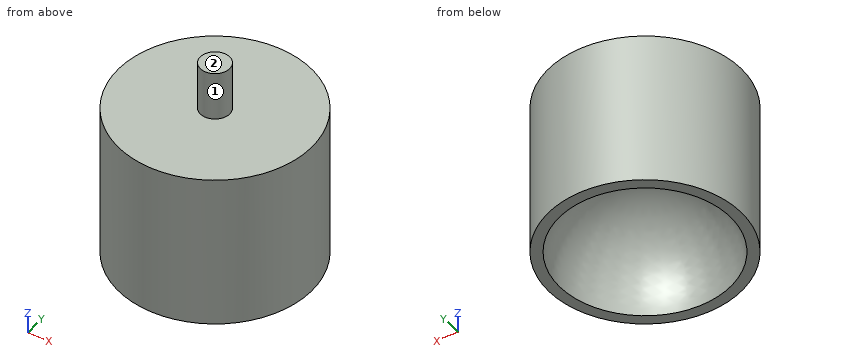
from build123d import *

# Parameters (mm, degrees)
F0_R     = 5.925
F1_DEPTH = 9.5
F2_R     = 0.9
F3_DEPTH = 3


with BuildPart() as f1:
    # F0 (on Top) → F1 (new body)
    with BuildSketch(Plane.XY):
        Circle(F0_R)
    extrude(amount=F1_DEPTH)

    # F2 (on face) → F3 (join)
    with BuildSketch(Plane.XY.offset(9.5)):
        Circle(F2_R)
    extrude(amount=F3_DEPTH)

    # F4 (on Front) → F5 (revolve, cut)
    with BuildSketch(Plane.XZ):
        with BuildLine():
            Line((0, 0), (5.25, 0))
            ThreePointArc((5.25, 0), (3.712311, 3.712311), (0, 5.25))
            Line((0, 5.25), (0, 0))
        make_face()
    revolve(axis=Axis((0, 0, 7.387147), (0, 0, 1)), mode=Mode.SUBTRACT)


solid = f1.part
Part model, mm, in its own coordinate system. Face numbers are marked on the shaded views. A direction names the side the tool comes from. Round coordinates to 2 decimals unless told otherwise and drop trailing zeros. Loops run counter-clockwise (first coordinate to the right, second up) from the corner with the lowest first, then second, coordinate; pieces in that order, holes last. Notation, with made-up numbers: (-3.5, 60.25) - (3.5, 60.25) arc R16 ccw to (3.5, 81.25) - close; hole circle Ø5 at (33, 54). An arc over 180 degrees is marked (long way). Answer as a JSON object with one key per item and string values.
Item 1: Band-saw the part on A-A on z = 6.5. List the corners of the cut face in (x, y) (3 decimals), plus the area to 3 significant figures.
Output:
{"outline": "circle Ø11.85 at (0, 0)", "area": "110 mm2"}
Item 2: Tool access for the marked faces 1 and 2: list every direction of +Z, -Z, +X, -X, +Y, -Y with a clear straight run to the whole face (end or side of a thin tool).
Output:
{"face 1": "+Z", "face 2": "+Z, +X, -X, +Y, -Y"}
Item 3: Pin check, flat tips, straight feed: pin 1 (2 mm diameter, centred on y = -3.5, z = 8, fed in from +X); pin 2 (4 mm diameter, centred on y = -2.5, z = 10.5, fed in from -X) (3 decimals); pin 3 (3 mm diameter, centred on x = 4.5, z = 9, fed in from +Y). Stop position of each tip, or through.
Output:
{"pin 1": "x = 5.37", "pin 2": "x = -5.875", "pin 3": "y = 5.11"}
Item 4: Wall check: L1, parallel to Z at x = -5, y = -2; L2, parallel to X at y = -2, z = 1; L3, parallel to Y at x = 3, z = 2. Give the ranges that are in metal, low to high.
Output:
{"L1": "0 to 9.5", "L2": "-5.58 to -4.75, 4.75 to 5.58", "L3": "-5.11 to -3.82, 3.82 to 5.11"}
